Check sheet for the modelled part. Datum: model origin and axes. Units: mm. Face numbers are marked on the shaded views. A direction names the side the tool comes from. Give positions to 0.01 mm unless a question says otherwise; leave off trailing zeros. Order: outer loops, then holes, each group sorted by start corner. A loop starts at its lowest first (then second) coordinate and runs counter-clockwise, first axis right, second up. Notation, with made-up numbers: (8, 45.5) -> (22, 45.5) arc R21 ccw to (22, 82.5) -> close; hole circle Ø4 at (-9, 84). An arc over 180 degrees is marked (long way). Write each question's results on one line, items separated by ' | '.
from build123d import *

# Parameters (mm, degrees)
SKETCH1_W           = 254
SKETCH1_H           = 127
BOSS_EXTRUDE2_DEPTH = 19.05
SKETCH2_W           = 244
SKETCH2_H           = 117
CUT_EXTRUDE1_DEPTH  = 17.05
SKETCH4_R           = 13
CUT_EXTRUDE2_DEPTH  = 17.05
SKETCH5_W           = 70
SKETCH5_H           = 127
CUT_EXTRUDE3_DEPTH  = 45
SKETCH6_W           = 5
SKETCH6_H           = 117
BOSS_EXTRUDE3_DEPTH = 17.05
BOSS_EXTRUDE4_START = 6
SKETCH7_W           = 184
SKETCH7_H           = 127
SKETCH7_R           = 13
BOSS_EXTRUDE4_DEPTH = 6
BOSS_EXTRUDE5_DEPTH = 17.05
SKETCH9_W           = 11.462803728
SKETCH9_H           = 5
BOSS_EXTRUDE6_DEPTH = 10
SKETCH10_R          = 1.5
CUT_EXTRUDE4_DEPTH  = 23
SKETCH11_W          = 5
SKETCH11_H          = 15
CUT_EXTRUDE6_DEPTH  = 1.5
SKETCH13_W          = 6.3
SKETCH13_H          = 6.3
CUT_EXTRUDE8_DEPTH  = 4.5
SKETCH16_R          = 1
CUT_EXTRUDE10_DEPTH = 5.5
SKETCH17_R          = 1.71
CUT_EXTRUDE11_DEPTH = 10


with BuildPart() as part:
    # Sketch1 → Boss-Extrude2 (new body)
    with BuildSketch(Plane(origin=(0, 0, 0), x_dir=(1, 0, 0), z_dir=(0, 1, 0))):
        Rectangle(SKETCH1_W, SKETCH1_H)
    extrude(amount=BOSS_EXTRUDE2_DEPTH)

    # Sketch2 → Cut-Extrude1 (cut)
    with BuildSketch(Plane.XZ):
        Rectangle(SKETCH2_W, SKETCH2_H)
    extrude(amount=-CUT_EXTRUDE1_DEPTH, mode=Mode.SUBTRACT)

    # Sketch4 → Cut-Extrude2 (cut)
    with BuildSketch(Plane(origin=(0, 19.05, 0), x_dir=(1, 0, 0), z_dir=(0, 1, 0))):
        with Locations(Location((92, 1.5, 0), (0, 0, 270))):
            Circle(SKETCH4_R)
        with Locations(Location((92, 31.5, 0), (0, 0, 270))):
            Circle(SKETCH4_R)
        with Locations(Location((62, 11.5, 0), (0, 0, 270))):
            Circle(SKETCH4_R)
        with Locations(Location((62, 41.5, 0), (0, 0, 270))):
            Circle(SKETCH4_R)
        with Locations(Location((32, 11.5, 0), (0, 0, 270))):
            Circle(SKETCH4_R)
        with Locations(Location((32, 41.5, 0), (0, 0, 270))):
            Circle(SKETCH4_R)
        with Locations(Location((2, -3.5, 0), (0, 0, 270))):
            Circle(SKETCH4_R)
        with Locations(Location((2, 26.5, 0), (0, 0, 270))):
            Circle(SKETCH4_R)
    extrude(amount=-CUT_EXTRUDE2_DEPTH, mode=Mode.SUBTRACT)

    # Sketch5 → Cut-Extrude3 (cut)
    with BuildSketch(Plane.XZ):
        with Locations((-92, 0)):
            Rectangle(SKETCH5_W, SKETCH5_H)
    extrude(amount=-CUT_EXTRUDE3_DEPTH, mode=Mode.SUBTRACT)

    # Sketch6 → Boss-Extrude3 (add)
    with BuildSketch(Plane.XZ.offset(-17.05)):
        with Locations((-54.5, 0)):
            Rectangle(SKETCH6_W, SKETCH6_H)
    extrude(amount=BOSS_EXTRUDE3_DEPTH)

    # Sketch7 → Boss-Extrude4 (add)
    with BuildSketch(Plane(origin=(0, 19.05, 0), x_dir=(1, 0, 0), z_dir=(0, 1, 0)).offset(BOSS_EXTRUDE4_START)):
        with Locations((35, 0)):
            Rectangle(SKETCH7_W, SKETCH7_H)
        with Locations(Location((2, 26.5, 0), (0, 0, 270))):
            Circle(SKETCH7_R, mode=Mode.SUBTRACT)
        with Locations(Location((2, -3.5, 0), (0, 0, 270))):
            Circle(SKETCH7_R, mode=Mode.SUBTRACT)
        with Locations(Location((32, 11.5, 0), (0, 0, 270))):
            Circle(SKETCH7_R, mode=Mode.SUBTRACT)
        with Locations(Location((92, 31.5, 0), (0, 0, 270))):
            Circle(SKETCH7_R, mode=Mode.SUBTRACT)
        with Locations(Location((62, 11.5, 0), (0, 0, 270))):
            Circle(SKETCH7_R, mode=Mode.SUBTRACT)
        with Locations(Location((62, 41.5, 0), (0, 0, 270))):
            Circle(SKETCH7_R, mode=Mode.SUBTRACT)
        with Locations(Location((32, 41.5, 0), (0, 0, 270))):
            Circle(SKETCH7_R, mode=Mode.SUBTRACT)
        with Locations(Location((92, 1.5, 0), (0, 0, 270))):
            Circle(SKETCH7_R, mode=Mode.SUBTRACT)
    extrude(amount=-BOSS_EXTRUDE4_DEPTH)

    # Sketch8 → Boss-Extrude5 (add)
    with BuildSketch(Plane.XZ.offset(-17.05)):
        with BuildLine():
            Line((118.5, 58.5), (122, 58.5))
            Line((122, 58.5), (122, 55))
            ThreePointArc((122, 55), (119.525126266, 56.025126266), (118.5, 58.5))
        make_face()
        with BuildLine():
            Line((122, -55), (122, -58.5))
            Line((122, -58.5), (118.5, -58.5))
            ThreePointArc((118.5, -58.5), (119.525126266, -56.025126266), (122, -55))
        make_face()
        with BuildLine():
            Line((-52, -55), (-52, -58.5))
            Line((-52, -58.5), (-48.5, -58.5))
            ThreePointArc((-48.5, -58.5), (-49.525126266, -56.025126266), (-52, -55))
        make_face()
        with BuildLine():
            Line((-52, 55), (-52, 58.5))
            Line((-52, 58.5), (-48.5, 58.5))
            ThreePointArc((-48.5, 58.5), (-49.525126266, 56.025126266), (-52, 55))
        make_face()
    extrude(amount=BOSS_EXTRUDE5_DEPTH)

    # Sketch9 → Boss-Extrude6 (add)
    with BuildSketch(Plane.XZ):
        with Locations((35, -61)):
            Rectangle(SKETCH9_W, SKETCH9_H)
    extrude(amount=BOSS_EXTRUDE6_DEPTH)

    # Sketch10 → Cut-Extrude4 (cut)
    with BuildSketch(Plane.XZ):
        with Locations(Location((122, -58.5, 0), (0, 0, 270))):
            Circle(SKETCH10_R)
        with Locations(Location((122, 58.5, 0), (0, 0, 270))):
            Circle(SKETCH10_R)
        with Locations(Location((-52, -58.5, 0), (0, 0, 270))):
            Circle(SKETCH10_R)
        with Locations(Location((-52, 58.5, 0), (0, 0, 270))):
            Circle(SKETCH10_R)
    extrude(amount=-CUT_EXTRUDE4_DEPTH, mode=Mode.SUBTRACT)

    # Sketch11 → Cut-Extrude6 (cut)
    with BuildSketch(Plane.XZ):
        with Locations((-54.5, -26)):
            Rectangle(SKETCH11_W, SKETCH11_H)
    extrude(amount=-CUT_EXTRUDE6_DEPTH, mode=Mode.SUBTRACT)

    # Sketch13 → Cut-Extrude8 (cut)
    with BuildSketch(Plane.XY.offset(-58.5)):
        with Locations((-30.184481008, 4.938954373)):
            Rectangle(SKETCH13_W, SKETCH13_H)
        with Locations((-40.184481008, 4.938954373)):
            Rectangle(SKETCH13_W, SKETCH13_H)
        with Locations((-20.184481008, 4.938954373)):
            Rectangle(SKETCH13_W, SKETCH13_H)
    extrude(amount=-CUT_EXTRUDE8_DEPTH, mode=Mode.SUBTRACT)

    # Sketch16 → Cut-Extrude10 (cut)
    with BuildSketch(Plane.XZ.offset(-17.05)):
        with Locations(Location((111.144556631, 25.062533315, 0), (0, 0, 270))):
            Circle(SKETCH16_R)
        with Locations(Location((111.144556631, -53.90768708, 0), (0, 0, 270))):
            Circle(SKETCH16_R)
        with Locations(Location((-23.950730393, -53.90768708, 0), (0, 0, 270))):
            Circle(SKETCH16_R)
        with Locations(Location((-23.950730393, 25.062533315, 0), (0, 0, 270))):
            Circle(SKETCH16_R)
    extrude(amount=-CUT_EXTRUDE10_DEPTH, mode=Mode.SUBTRACT)

    # Sketch17 → Cut-Extrude11 (cut)
    with BuildSketch(Plane.XY.offset(-63)):
        with Locations((-40.184481008, 4.938954373)):
            Circle(SKETCH17_R)
        with Locations((-30.184481008, 4.938954373)):
            Circle(SKETCH17_R)
        with Locations((-20.184481008, 4.938954373)):
            Circle(SKETCH17_R)
    extrude(amount=-CUT_EXTRUDE11_DEPTH, mode=Mode.SUBTRACT)


solid = part.part
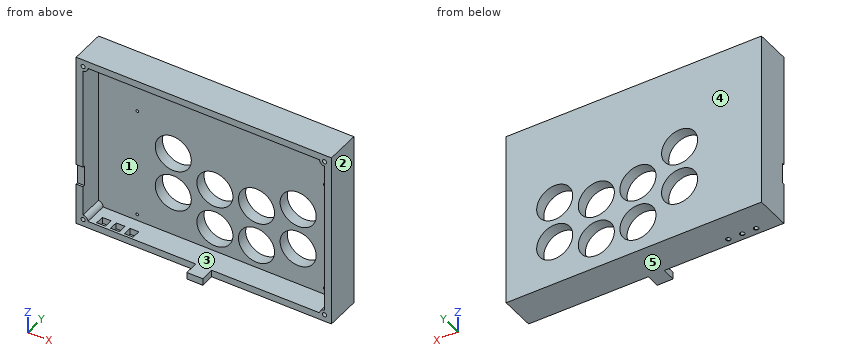
1. Material ranges on probe 1 along Z at (x, y) = (82.5, 16); probe 2 along X at (y, z) = (7, -20); probe 3 along X at (y, z) = (20, -1), recorded low to high. Write a range as from..to.
Verdict:
probe 1: z = -63.5..-58.5, 58.5..63.5 | probe 2: x = -57..-52, 122..127 | probe 3: x = -57..-10.2, 14.2..24.34, 39.66..54.34, 69.66..79.01, 104.99..127
2. Section check D-D on y = -7. Record the cut outline in (x, z), then the cut area to 3 significant figures.
Verdict:
outline: (29.27, -63.5) -> (40.73, -63.5) -> (40.73, -58.5) -> (29.27, -58.5) -> close | area: 57.3 mm^2
3. Gauge pin test, flat ends, axial feed: pin 1 Ø1.5 at (x, z) = (55, 8) entering from -Y; pin 2 Ø1.8 at (x, z) = (122, 58.5) entering from -Y; pin 3 Ø2.5 at (x, y) = (-20.18, 4.94) entering from -Z. Record the tip position at first contact, or that the pin passes through.
Verdict:
pin 1: stops at y = 17.05 | pin 2: stops at y = 23 | pin 3: stops at z = 58.5
4. Mould release check, pull along Z, two halves, no side actions. Record for the marked faces 3, 4 and 5: +Z half, -Z half, draft (parallel to the pull), parting line (faces both ways), or undercut.
Verdict:
face 3: undercut | face 4: draft | face 5: -Z half
5. Access from +Z, -Z, +X, -X, +Y, -Y to the whole of each face (thin tool, end or side, straight path). Record for the marked faces 1 and 2.
Verdict:
face 1: -Y | face 2: +Z, -Z, +X, +Y, -Y
6. Section check C-C on z = 41. Record the cut outline in (x, y).
Verdict:
outline: (-57, 0) -> (-52, 0) -> (-52, 17.05) -> (122, 17.05) -> (122, 0) -> (127, 0) -> (127, 25.05) -> (-57, 25.05) -> close
7. Section check A-A on x = 92. Record the cut outline in (y, z), then the cut area to 4 significant figures.
Verdict:
outline: (0, -63.5) -> (25.05, -63.5) -> (25.05, -44.5) -> (17.05, -44.5) -> (17.05, -58.5) -> (0, -58.5) -> close; (0, 58.5) -> (17.05, 58.5) -> (17.05, 11.5) -> (25.05, 11.5) -> (25.05, 63.5) -> (0, 63.5) -> close; (17.05, -18.5) -> (25.05, -18.5) -> (25.05, -14.5) -> (17.05, -14.5) -> close | area: 770.5 mm^2
8. Section check B-B on z = -26.5. Record the cut outline in (x, y).
Verdict:
outline: (-57, 1.5) -> (-52, 1.5) -> (-52, 17.05) -> (-11, 17.05) -> (-11, 25.05) -> (-57, 25.05) -> close; (15, 17.05) -> (80, 17.05) -> (80, 25.05) -> (15, 25.05) -> close; (104, 17.05) -> (122, 17.05) -> (122, 0) -> (127, 0) -> (127, 25.05) -> (104, 25.05) -> close
